```python
from build123d import *

# Parameters (mm, degrees)
SKETCH12_R              = 16
BOSS_EXTRUDE3_DEPTH     = 5
CUT_EXTRUDE3_REACH      = 25.173
SKETCH14_R              = 2.4
BOSS_EXTRUDE4_DEPTH     = 8
SKETCH15_R              = 5.25
CUT_EXTRUDE4_DEPTH      = 10
CUT_EXTRUDE5_REACH      = 31.335
CUT_EXTRUDE5_END_RADIUS = 5.25
SKETCH17_R              = 2.4


with BuildPart() as part:
    # Sketch12 → Boss-Extrude3 (new body)
    with BuildSketch(Plane.XY):
        Circle(SKETCH12_R)
    extrude(amount=BOSS_EXTRUDE3_DEPTH)

    # Sketch14 → Cut-Extrude3 (cut, up to next)
    with BuildSketch(Plane.XY, mode=Mode.PRIVATE) as cut_extrude3_sk1:
        with Locations((8.838834765, 8.838834765)):
            Circle(SKETCH14_R)
    cut_extrude3_tool1 = extrude(cut_extrude3_sk1.sketch, amount=CUT_EXTRUDE3_REACH, mode=Mode.PRIVATE) & part.part
    # Sketch14 → Cut-Extrude3 (cut, up to next)
    with BuildSketch(Plane.XY, mode=Mode.PRIVATE) as cut_extrude3_sk2:
        with Locations((-8.838834765, 8.838834765)):
            Circle(SKETCH14_R)
    cut_extrude3_tool2 = extrude(cut_extrude3_sk2.sketch, amount=CUT_EXTRUDE3_REACH, mode=Mode.PRIVATE) & part.part
    # Sketch14 → Cut-Extrude3 (cut, up to next)
    with BuildSketch(Plane.XY, mode=Mode.PRIVATE) as cut_extrude3_sk3:
        with Locations((8.838834765, -8.838834765)):
            Circle(SKETCH14_R)
    cut_extrude3_tool3 = extrude(cut_extrude3_sk3.sketch, amount=CUT_EXTRUDE3_REACH, mode=Mode.PRIVATE) & part.part
    # Sketch14 → Cut-Extrude3 (cut, up to next)
    with BuildSketch(Plane.XY, mode=Mode.PRIVATE) as cut_extrude3_sk4:
        with Locations((-8.838834765, -8.838834765)):
            Circle(SKETCH14_R)
    cut_extrude3_tool4 = extrude(cut_extrude3_sk4.sketch, amount=CUT_EXTRUDE3_REACH, mode=Mode.PRIVATE) & part.part
    add(cut_extrude3_tool1.solids().sort_by_distance((8.838835, 8.838835, 0))[0], mode=Mode.SUBTRACT)
    add(cut_extrude3_tool2.solids().sort_by_distance((-8.838835, 8.838835, 0))[0], mode=Mode.SUBTRACT)
    add(cut_extrude3_tool3.solids().sort_by_distance((8.838835, -8.838835, 0))[0], mode=Mode.SUBTRACT)
    add(cut_extrude3_tool4.solids().sort_by_distance((-8.838835, -8.838835, 0))[0], mode=Mode.SUBTRACT)

    # Sketch16 → Boss-Extrude4 (add)
    with BuildSketch(Plane.XY):
        with BuildLine():
            Line((4, 7.25), (-4, 7.25))
            ThreePointArc((-4, 7.25), (0, -8.280247581), (4, 7.25))
        make_face()
    extrude(amount=-BOSS_EXTRUDE4_DEPTH)

    # Sketch15 → Cut-Extrude4 (cut, symmetric)
    with BuildSketch(Plane.XY):
        Circle(SKETCH15_R)
    extrude(amount=CUT_EXTRUDE4_DEPTH, both=True, mode=Mode.SUBTRACT)

    # Cut-Extrude5: up to this cylinder (the profile starts outside it)
    cut_extrude5_end = Plane(origin=(0, 0, -4), z_dir=(0, 0, 1)) * Cylinder(CUT_EXTRUDE5_END_RADIUS, 74.17, mode=Mode.PRIVATE)
    # Sketch17 → Cut-Extrude5 (cut, up to the surface)
    with BuildSketch(Plane(origin=(0, 7.25, 0), x_dir=(1, 0, 0), z_dir=(0, 1, 0)), mode=Mode.PRIVATE) as cut_extrude5_sk1:
        with Locations(Location((0, 4, 0), (0, 0, 270))):
            Circle(SKETCH17_R)
    cut_extrude5_tool1 = extrude(cut_extrude5_sk1.sketch, amount=-CUT_EXTRUDE5_REACH, mode=Mode.PRIVATE) - cut_extrude5_end
    add(cut_extrude5_tool1.solids().sort_by_distance((0, 7.25, -4))[0], mode=Mode.SUBTRACT)


solid = part.part
```
Model file for the job. Use its own axes, mm. A direction names the side the tool comes from. Round coordinates to 2 decimals unless told otherwise and drop trailing zeros. Loops run counter-clockwise (first coordinate to the right, second up) from the corner with the lowest first, then second, coordinate; pieces in that order, holes last. Notation, with made-up numbers: M 62,-17.5 L 91,-17.5 A36 ccw 91,16.5 Z; hole C 3.5,-23 d1. An arc over 180 degrees is marked long. Put each result on its own line as item: value. Start each with the question number.
Item 1: 3-axis set-ups, long thin cutter, end or side, ignore diameter. For faces 5 (the face through (-10.61, 10.46, 2.46)), 6 (the face through (-1.46, 5.978, -5.905)), 7 (the face through (7, 7, 0)): which of +Z, -Z, +X, -X, +Y, -Y reach the whole face in a straight line?
Item 2: Drill centre lines: line 1 along X through (y, z) = (-8, 0.75); line 2 along Y through (x, z) = (-7, 4); line 3 along Z through (x, y) = (0, 5.6). Where is each one in solid material? Low to high.
Item 3: Cut at D-D (z = 2.25). List the corners of the cut face in (x, y).
Item 4: Drop flat-ended pins along their axis: P1, Ø4, axis at x = 8.84, y = 8.84, coming from the -Z side; P2, Ø2.5, axis at x = -1.5, z = -2.5, coming from the +Y side; P3, Ø2, axis at x = -8, z = 1.5, coming from the +Y side; P4, Ø2, axis at y = -8, z = -1.5, coming from the +X side. Give the stop position or say it passes through.
Item 5: Cut at B-B (y = 0). List the corners of the cut face in (x, z).
Item 6: Cut at A-A (x = 0). List the corners of the cut face in (y, z), then the cut area to 3 significant figures.
Item 7: Mould opens along Y. For faces 1 (the face through (-0.306, -8.275, -3.944)), 2 (the face through (8.53, 11.22, 2.46)), 3 (the face through (2, 7.25, -6)), 4 (the face through (4, -4, -8)) say: released by +Y, released by -Y, zero draft, split by the parting line, or undercut.
Item 8: Cut at C-C (z = -4). List the corners of the cut face in (x, y), then the cut area to 3 significant figures.
Answer block:
1. face 5: +Z, -Z
1. face 6: +Y
1. face 7: -Z
2. line 1: -13.86 to -11.09, -6.59 to 6.59, 11.09 to 13.86
2. line 2: -14.39 to -10.38, -7.3 to 7.3, 10.38 to 14.39
2. line 3: -8 to -6.4, -1.6 to 5
3. outline: C 0,0 d32; hole C -8.84,-8.84 d4.8; hole C -8.84,8.84 d4.8; hole C 0,0 d10.5; hole C 8.84,-8.84 d4.8; hole C 8.84,8.84 d4.8
4. P1: through
4. P2: y = 7.25
4. P3: y = 14.39
4. P4: x = 4.42
5. outline: M -16,0 L -8.28,0 L -8.28,-8 L -5.25,-8 L -5.25,5 L -16,5 Z; M 5.25,-8 L 8.28,-8 L 8.28,0 L 16,0 L 16,5 L 5.25,5 Z
6. outline: M -16,0 L -8.28,0 L -8.28,-8 L -5.25,-8 L -5.25,5 L -16,5 Z; M 5.25,-8 L 7.25,-8 L 7.25,-6.4 L 5.25,-6.4 Z; M 5.25,-1.6 L 7.25,-1.6 L 7.25,0 L 16,0 L 16,5 L 5.25,5 Z
6. area: 138 mm2
7. face 1: split by the parting line
7. face 2: undercut
7. face 3: released by +Y
7. face 4: zero draft
8. outline: M -4,7.25 A8.28 ccw long 4,7.25 L 2.4,7.25 L 2.4,4.67 A5.25 cw long -2.4,4.67 L -2.4,7.25 Z
8. area: 113 mm2
